For this review, use the dimensioned drawing (mm, ordinates from the lowest corner) and the shaded views. A direction names the side the tool comes from. Round coordinates to 2 decimals unless told otherwise and drop trailing zeros. Loops run counter-clockwise (first coordinate to the right, second up) from the corner with the lowest first, then second, coordinate; pieces in that order, holes last. Notation, with made-up numbers: M -13,85 L 1,85 A33 ccw 1,117 Z; hole C 88,31.25 d2. An arc over 180 degrees is marked long. One line per item, written item: value. Start each with the question number.
Item 1: Clearance check with flat-ended pins moving along their axes: pin 1 (10 mm diameter, centred on x = 105.5, z = 51.5, fed in from -Y); pin 2 (1 mm diameter, centred on x = 112, z = 15.5, fed in from +Y); pin 3 (12 mm diameter, centred on x = 117.5, y = 89.5, fed in from +Z); pin 4 (20.5 mm diameter, centred on x = 22.48, y = 50.8, fed in from +Z). State where each tip first meets the part, or that it passes through.
Item 2: We need section D-D (y = 21). Write out the cut boundary in (x, z) (1 decimal), then the cut area to 3 significant figures.
Item 3: We need section A-A (y = 50.8). Write out the cut boundary in (x, z) (1 decimal).
Item 4: For the marked faces 1, 2 and 3, list the 3-axis set-ups (+Z, -Z, +X, -X, +Y, -Y) from which the entire face can be reached by the end or side of a thin tool; tool diameter is ignored.
Item 5: Mouldability with a two-part tool opening along X and no side actions: class the marked faces 4, 5 and 6 as released by +X, released by -X, zero draft, split by the parting line, or undercut.
Item 6: We need section C-C (z = 35). Write out the cut boundary in (x, y).
Item 7: For line 1 along X through (y, z) = (50, 34); line 2 along Y through (x, z) = (32.5, 74.5); line 3 along Y through (x, z) = (71, 14), list the stretches that pass through material, from the lowest coordinate up.
Item 8: We need section B-B (x = 18.5). Write out the cut boundary in (y, z).
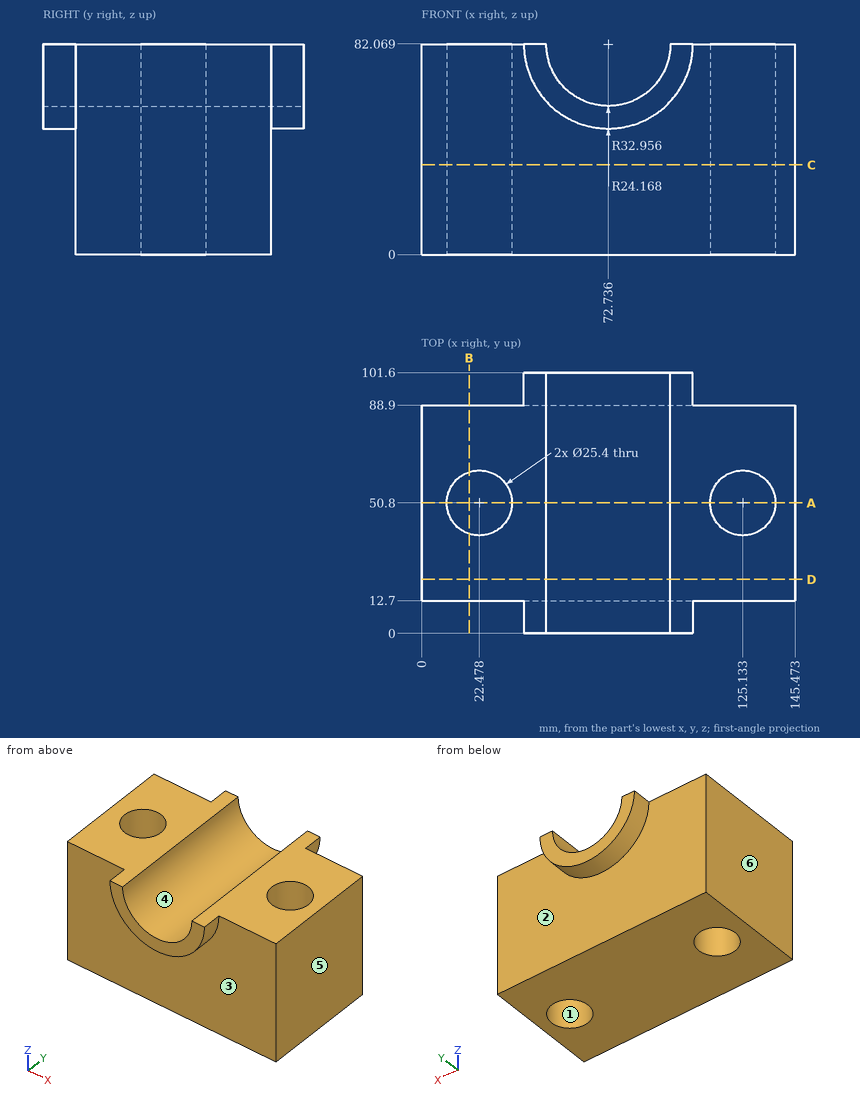
A:
1. pin 1: y = 12.7
1. pin 2: y = 88.9
1. pin 3: z = 82.07
1. pin 4: through
2. outline: M 0,0 L 145.5,0 L 145.5,82.1 L 96.9,82.1 A24.2 cw 48.6,82.1 L 0,82.1 Z
2. area: 11,000 mm2
3. outline: M 0,0 L 9.8,0 L 9.8,82.1 L 0,82.1 Z; M 35.2,0 L 112.4,0 L 112.4,82.1 L 96.9,82.1 A24.2 cw 48.6,82.1 L 35.2,82.1 Z; M 137.8,0 L 145.5,0 L 145.5,82.1 L 137.8,82.1 Z
4. face 1: +Z, -Z
4. face 2: -Z, +Y
4. face 3: -Z, -Y
5. face 4: undercut
5. face 5: released by +X
5. face 6: released by -X
6. outline: M 0,12.7 L 145.47,12.7 L 145.47,88.9 L 0,88.9 Z; hole C 22.48,50.8 d25.4; hole C 125.13,50.8 d25.4
7. line 1: 0 to 9.8, 35.15 to 112.46, 137.81 to 145.47
7. line 2: 12.7 to 43, 58.6 to 88.9
7. line 3: 12.7 to 88.9
8. outline: M 12.7,0 L 38.74,0 L 38.74,82.07 L 12.7,82.07 Z; M 62.86,0 L 88.9,0 L 88.9,82.07 L 62.86,82.07 Z
